```python
from build123d import *

# Parameters (mm, degrees)
SKETCH1_R           = 2.5
BOSS_EXTRUDE1_DEPTH = 1.5
BOSS_EXTRUDE2_DEPTH = 3.5


with BuildPart() as part:
    # Sketch1 → Boss-Extrude1 (new body)
    with BuildSketch(Plane.XY):
        with BuildLine():
            Line((39, 20), (-39, 20))
            ThreePointArc((-39, 20), (-39.707106781, 19.707106781), (-40, 19))
            Line((-40, 19), (-40, -19))
            ThreePointArc((-40, -19), (-39.707106781, -19.707106781), (-39, -20))
            Line((-39, -20), (39, -20))
            ThreePointArc((39, -20), (39.707106781, -19.707106781), (40, -19))
            Line((40, -19), (40, 19))
            ThreePointArc((40, 19), (39.707106781, 19.707106781), (39, 20))
        make_face()
        with Locations((-36, 16)):
            Circle(SKETCH1_R, mode=Mode.SUBTRACT)
        with Locations((-36, -16)):
            Circle(SKETCH1_R, mode=Mode.SUBTRACT)
        with Locations(Location((36, -16, 0), (0, 0, 180))):
            Circle(SKETCH1_R, mode=Mode.SUBTRACT)
        with Locations(Location((36, 16, 0), (0, 0, 180))):
            Circle(SKETCH1_R, mode=Mode.SUBTRACT)
        with BuildLine():
            Line((26.244997998, 19), (-26.244997998, 19))
            ThreePointArc((-26.244997998, 19), (-28.977515605, 17.871883325), (-31.513890212, 16.353297288))
            ThreePointArc((-31.513890212, 16.353297288), (-32.818019485, 12.818019485), (-36.353297288, 11.513890212))
            ThreePointArc((-36.353297288, 11.513890212), (-37.871883325, 8.977515605), (-39, 6.244997998))
            Line((-39, 6.244997998), (-39, -6.244997998))
            ThreePointArc((-39, -6.244997998), (-37.871883325, -8.977515605), (-36.353297288, -11.513890212))
            ThreePointArc((-36.353297288, -11.513890212), (-32.818019485, -12.818019485), (-31.513890212, -16.353297288))
            ThreePointArc((-31.513890212, -16.353297288), (-28.977515605, -17.871883325), (-26.244997998, -19))
            Line((-26.244997998, -19), (26.244997998, -19))
            ThreePointArc((26.244997998, -19), (28.977515605, -17.871883325), (31.513890212, -16.353297288))
            ThreePointArc((31.513890212, -16.353297288), (32.818019485, -12.818019485), (36.353297288, -11.513890212))
            ThreePointArc((36.353297288, -11.513890212), (37.871883325, -8.977515605), (39, -6.244997998))
            Line((39, -6.244997998), (39, 6.244997998))
            ThreePointArc((39, 6.244997998), (37.871883325, 8.977515605), (36.353297288, 11.513890212))
            ThreePointArc((36.353297288, 11.513890212), (32.818019485, 12.818019485), (31.513890212, 16.353297288))
            ThreePointArc((31.513890212, 16.353297288), (28.977515605, 17.871883325), (26.244997998, 19))
        make_face(mode=Mode.SUBTRACT)
    extrude(amount=BOSS_EXTRUDE1_DEPTH)

    # Sketch2 → Boss-Extrude2 (add)
    with BuildSketch(Plane(origin=(0, 0, 0), x_dir=(-1, 0, 0), z_dir=(0, 0, -1))):
        with BuildLine():
            Line((39, 22), (-39, 22))
            ThreePointArc((-39, 22), (-41.121320344, 21.121320344), (-42, 19))
            Line((-42, 19), (-42, -19))
            ThreePointArc((-42, -19), (-41.121320344, -21.121320344), (-39, -22))
            Line((-39, -22), (39, -22))
            ThreePointArc((39, -22), (41.121320344, -21.121320344), (42, -19))
            Line((42, -19), (42, 19))
            ThreePointArc((42, 19), (41.121320344, 21.121320344), (39, 22))
        make_face()
        with BuildLine():
            Line((40, -19), (40, 19))
            ThreePointArc((40, 19), (39.707106781, 19.707106781), (39, 20))
            Line((39, 20), (-39, 20))
            ThreePointArc((-39, 20), (-39.707106781, 19.707106781), (-40, 19))
            Line((-40, 19), (-40, -19))
            ThreePointArc((-40, -19), (-39.707106781, -19.707106781), (-39, -20))
            Line((-39, -20), (39, -20))
            ThreePointArc((39, -20), (39.707106781, -19.707106781), (40, -19))
        make_face(mode=Mode.SUBTRACT)
    extrude(amount=-BOSS_EXTRUDE2_DEPTH)


solid = part.part
```
Could you check a few things on this model? Use its own coordinates, in mm. A direction names the side the tool comes from. Give positions to 0.01 mm unless a question says otherwise; leave off trailing zeros. Order: outer loops, then holes, each group sorted by start corner. A loop starts at its lowest first (then second) coordinate and runs counter-clockwise, first axis right, second up.
Q1. We'd pull the mould along X, two halves only. Please class faces 1 (the flat face through (-42, 0, 2)), 2 (the flat face through (42, 0, 2)), 3 (the cylindrical face through (32.78, -12.857, 0.74)): +X half, -X half, draft (parallel to the pull), parting line (faces both ways), or undercut.
Q2. For faces 4 (the cylindrical face through (32.857, 12.78, 0.74)), 5 (the flat face through (-1, 22, 2)), 6 (the flat face through (40, 0, 2)), which set-ups out of +Z, -Z, +X, -X, +Y, -Y let a thin tool reach every point of the face, with its end or its side?
Q3. Suppose I cut it at A-A, the plane x = -0.5. Write out the boundary of the cut face in (y, z), and give its area (3 significant figures).
Q4. I'm going to push a flat-ended pin straight in: P1, Ø4.5, axis at x = -36, y = 16, coming from the -Z side. Where does the tip first touch, or does it pass through?
Q5. Suppose I cut it at C-C, the plane z = 0.85. Write out the boundary of the cut face in (x, y) (3 decimals).
Q6. Suppose I cut it at B-B, the plane y = -8. Write out the boundary of the cut face in (x, z), and give its area (3 significant figures).
Q7. If I drill on line 1 along Y through (x, z) = (-36, 0.65); line 2 along X through (y, z) = (14, 2); line 3 along Y through (x, z) = (-18.5, 1.95), over which ranges is the centre line in solid material (lowest first)?
Q8. Suppose I cut it at D-D, the plane y = -14.5. Write out the boundary of the cut face in (x, z).
Solution:
1. face 1: -X half
1. face 2: +X half
1. face 3: undercut
2. face 4: +Z, -Z
2. face 5: +Z, -Z, +X, -X, +Y
2. face 6: +Z
3. outline: (-22, 0) - (-19, 0) - (-19, 1.5) - (-20, 1.5) - (-20, 3.5) - (-22, 3.5) - close; (19, 0) - (22, 0) - (22, 3.5) - (20, 3.5) - (20, 1.5) - (19, 1.5) - close
3. area: 17.0 mm2
4. P1: passes through
5. outline: (-42, -19) arc R3 ccw to (-39, -22) - (39, -22) arc R3 ccw to (42, -19) - (42, 19) arc R3 ccw to (39, 22) - (-39, 22) arc R3 ccw to (-42, 19) - close; hole (-39, -6.245) arc R20 ccw to (-36.353, -11.514) arc R4.5 cw to (-31.514, -16.353) arc R20 ccw to (-26.245, -19) - (26.245, -19) arc R20 ccw to (31.514, -16.353) arc R4.5 cw to (36.353, -11.514) arc R20 ccw to (39, -6.245) - (39, 6.245) arc R20 ccw to (36.353, 11.514) arc R4.5 cw to (31.514, 16.353) arc R20 ccw to (26.245, 19) - (-26.245, 19) arc R20 ccw to (-31.514, 16.353) arc R4.5 cw to (-36.353, 11.514) arc R20 ccw to (-39, 6.245) - close; hole circle Ø5 at (-36, -16); hole circle Ø5 at (-36, 16); hole circle Ø5 at (36, -16); hole circle Ø5 at (36, 16)
6. outline: (-42, 0) - (-38.33, 0) - (-38.33, 1.5) - (-40, 1.5) - (-40, 3.5) - (-42, 3.5) - close; (38.33, 0) - (42, 0) - (42, 3.5) - (40, 3.5) - (40, 1.5) - (38.33, 1.5) - close
6. area: 19.0 mm2
7. line 1: y = -22 to -18.5, -13.5 to -11.5, 11.5 to 13.5, 18.5 to 22
7. line 2: x = -42 to -40, 40 to 42
7. line 3: y = -22 to -20, 20 to 22
8. outline: (-42, 0) - (-38, 0) - (-38, 1.5) - (-40, 1.5) - (-40, 3.5) - (-42, 3.5) - close; (-34, 0) - (-31.76, 0) - (-31.76, 1.5) - (-34, 1.5) - close; (31.76, 0) - (34, 0) - (34, 1.5) - (31.76, 1.5) - close; (38, 0) - (42, 0) - (42, 3.5) - (40, 3.5) - (40, 1.5) - (38, 1.5) - close
